CAD build for the part. Positions are in the model's coordinates, mm. Face numbers are marked on the shaded views. A direction names the side the tool comes from. Give positions to 0.01 mm unless a question says otherwise; leave off trailing zeros. Order: outer loops, then holes, each group sorted by start corner. A loop starts at its lowest first (then second) coordinate and runs counter-clockwise, first axis right, second up. Notation, with made-up numbers: M 51.25,51 L 97.25,51 A32 cw 97.25,87 Z; hole C -15,57.25 d9. An arc over 180 degrees is marked long. Put each result on its own line as item: value. Start each with the question number.
1) Cut at B-B (z = 2.8). Write the cut outline in (x, y).
2) Two-plate mould, pull along Y, no slides. Class the marked faces 1, 2 and 3: released by +Y, released by -Y, zero draft, split by the parting line, or undercut.
3) Tool access for the marked faces 4, 5 and 6: list every direction of +Z, -Z, +X, -X, +Y, -Y with a clear straight run to the whole face (end or side of a thin tool).
4) Cut at A-A (y = 7). Write the cut outline in (x, z).
5) Cut at D-D (x = 6.5). Write the cut outline in (y, z).
6) Drill centre lines: line 1 (Y direction, x = 13, z = 0.75); line 2 (X direction, y = 10.5, z = 4.6); line 3 (Y direction, x = 11, z = 3.3). Where is each one in solid material? Low to high. Write a range as [from, to].
7) Pin check, flat tips, straight feed: pin 1 (1 mm diameter, centred on x = -10.5, z = 0.5, fed in from -Y); pin 2 (9.5 mm diameter, centred on x = -13.86, y = -1.09, fed in from +Z). Stop position of each tip, or through.
8) Cut at C-C (y = -1.5). Write the cut outline in (x, z), and give its area (3 significant figures).
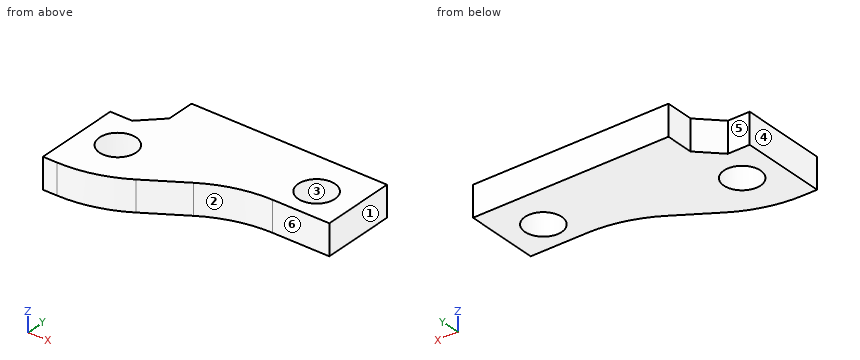
Autodesk Inventor part; units mm, degrees
ref_plane "YZ Plane" through (0, 0, 0) normal (1, 0, 0) x (0, 1, 0)
ref_plane "XZ Plane" through (0, 0, 0) normal (0, 1, 0) x (-1, 0, 0)
ref_plane "XY Plane" through (0, 0, 0) normal (0, 0, 1) x (1, 0, 0)
sketch "草图1" plane through (0, 0, 0) normal (0, 0, 1) x (1, 0, 0)
  line L0 (3.3485, 1.7155) -> (3.3485, -8.2845)
  line L1 (3.3485, -8.2845) -> (-18.6515, -8.2845)
  line L2 (-18.6515, -8.2845) -> (-18.6515, 3.7155)
  line L3 (-18.6515, 3.7155) -> (-15.6515, 3.7155)
  line L4 (-11.6515, 7.7155) -> (-15.6515, 3.7155)
  line L5 (-11.6515, 11.7155) -> (-11.6515, 7.7155)
  line L6 (18.3485, 11.7155) -> (-11.6515, 11.7155)
  line L7 (18.3485, 1.7155) -> (18.3485, 11.7155)
  line L8 (18.3485, 1.7155) -> (3.3485, 1.7155)
  circle A0 centre (13.2421, 5.8327) radius 3
  circle A1 centre (-13.8563, -1.088) radius 3
  line L9 (-12.6515, 12.7155) -> (-12.6515, 8.1297)
  line L10 (-12.6515, 8.1297) -> (-16.0657, 4.7155)
  line L11 (-16.0657, 4.7155) -> (-19.6515, 4.7155)
  line L12 (-19.6515, 4.7155) -> (-19.6515, -9.2845)
  line L13 (-19.6515, -9.2845) -> (4.3485, -9.2845)
  line L14 (4.3485, -9.2845) -> (4.3485, 0.7155)
  line L15 (4.3485, 0.7155) -> (19.3485, 0.7155)
  line L16 (19.3485, 0.7155) -> (19.3485, 12.7155)
  line L17 (19.3485, 12.7155) -> (-12.6515, 12.7155)
  dimension "d2" = 1
extrude "拉伸1" add sketch "草图1" along normal blind 5 contours L0 L1 L2 L3 L4 L5 L6 L7 L8 | L17 L16 L15 L14 L13 L12 L11 L10 L9
sketch "草图2" plane through (0, 0, 0) normal (0, 0, -1) x (-1, 0, 0)
  line L0 (3.2234, -5.6845) -> (-9.038, -5.6845)
  arc A0 (6.2234, -8.6845) -> (3.2234, -5.6845) centre (3.2234, -8.6845) ccw
  line L1 (-4.3485, -9.2845) -> (-4.3485, 0.7155)
  line L2 (-4.3485, 0.7155) -> (11.6515, -9.2845)
  line L3 (19.6515, -9.2845) -> (-4.3485, -9.2845)
  line L4 (19.6515, 4.7155) -> (19.6515, -9.2845)
  point P0 (0, 0)
  dimension "d5" = 8
extrude "拉伸2" cut sketch "草图2" against normal blind 5
fillet "圆角1" radius 20 2 edges at (4.3485, 0.7155, 2.5) (-11.6515, -9.2845, 2.5)
properties part number "阻挡X轴"
Solution:
1. outline: M -19.65,-9.28 L -17.39,-9.28 A20 ccw -6.79,-6.24 L -0.52,-2.32 A20 cw 10.08,0.72 L 19.35,0.72 L 19.35,12.72 L -12.65,12.72 L -12.65,8.13 L -16.07,4.72 L -19.65,4.72 Z; hole C -13.86,-1.09 d6; hole C 13.24,5.83 d6
2. face 1: zero draft
2. face 2: released by -Y
2. face 3: undercut
3. face 4: +Z, -Z, -X, +Y, -Y
3. face 5: +Z, -Z, -X, +Y
3. face 6: +Z, -Z, +X, -Y
4. outline: M -13.78,0 L 10.48,0 L 10.48,5 L -13.78,5 Z; M 16.01,0 L 19.35,0 L 19.35,5 L 16.01,5 Z
5. outline: M 0.39,0 L 12.72,0 L 12.72,5 L 0.39,5 Z
6. line 1: [0.72, 2.84], [8.82, 12.72]
6. line 2: [-12.65, 19.35]
6. line 3: [0.72, 3.84], [7.83, 12.72]
7. pin 1: y = -8.24
7. pin 2: z = 5
8. outline: M -19.65,0 L -16.83,0 L -16.83,5 L -19.65,5 Z; M -10.88,0 L 0.94,0 L 0.94,5 L -10.88,5 Z
8. area: 73.2 mm²
